The model under review builds one solid part; all positions refer to its coordinate system, in mm. Round coordinates to 2 decimals unless told otherwise and drop trailing zeros. Write each loop counter-clockwise with the first axis right and the second up, starting at its lowest first coordinate (ties: lowest second). Pieces come first, ordered by that corner, then holes. Notation, with made-up numbers: (78, 74.25) - (108, 74.25) arc R21 ccw to (108, 80.25) - close; hole circle Ø11 at (51.5, -11.5). An arc over 180 degrees is marked (long way). Return JSON: item names as keys, results as strings.
Autodesk Inventor part; units mm, degrees
ref_plane "CP_XY" through (0, 0, 0) normal (1, 0, 0) x (0, 0, -1)
ref_plane "CP_YZ" through (0, 0, 0) normal (0, 0, -1) x (0, 1, 0)
ref_plane "CP_ZX" through (0, 0, 0) normal (0, 1, 0) x (1, 0, 0)
sketch "Sketch_1" plane through (0, 0, 0) normal (0, 0, 1) x (1, 0, 0)
  line L0 (0, 0) -> (-4, 0)
  line L1 (-4, 0) -> (-4, 2.0095)
  line L2 (-4, 2.0095) -> (-3.5095, 2.5)
  line L3 (-3.5095, 2.5) -> (-0.75, 2.5)
  line L4 (-0.75, 2.5) -> (0, 1.75)
  line L5 (0, 1.75) -> (0, 0)
  line L6 (0, 0) -> (-4, 0)
revolve "Revolution1" add sketch "Sketch_1" angle 360 about axis through (0, 0, 0) along (1, 0, 0)
thread "Thread1"
sketch "Sketch_2" plane through (-4, 0, 0) normal (-1, 0, 0) x (0, 1, 0)
  line L0 (-1.25, 0.7217) -> (-1.25, -0.7217)
  line L1 (-1.25, -0.7217) -> (0, -1.4434)
  line L2 (0, -1.4434) -> (1.25, -0.7217)
  line L3 (1.25, -0.7217) -> (1.25, 0.7217)
  line L4 (1.25, 0.7217) -> (0, 1.4434)
  line L5 (0, 1.4434) -> (-1.25, 0.7217)
extrude "Extrusion1" cut sketch "Sketch_2" against normal blind 2
sketch "Sketch_3" plane through (0, 0, 0) normal (0, 0, 1) x (1, 0, 0)
  line L0 (-1.2783, 0) -> (-2, 0)
  line L1 (-2, 0) -> (-2, 1.25)
  line L2 (-2, 1.25) -> (-1.2783, 0)
  line L3 (-1.2783, 0) -> (-2, 0)
revolve "Revolution2" cut sketch "Sketch_3" angle 360 about axis through (-1.2783, 0, 0) along (1, 0, 0)
ref_plane "CP_XY" through (0, 0, 0) normal (1, 0, 0) x (0, 0, -1)
ref_plane "CP_YZ" through (0, 0, 0) normal (0, 0, -1) x (0, 1, 0)
ref_plane "CP_ZX" through (0, 0, 0) normal (0, 1, 0) x (1, 0, 0)
properties part number "SET-SCREW5-4"
(1) Mouldability with a two-part tool opening along Y and no side actions: class faces 1 (the cylindrical face through (-2.11, -0.54, -2.44)), 2 (the flat face through (-3.01, 0.63, -1.08)), 3 (the flat face through (0, 0, 0)) as released by +Y, released by -Y, zero draft, split by the parting line, or undercut.
Filled in:
{"face 1": "split by the parting line", "face 2": "undercut", "face 3": "zero draft"}
(2) Add section C-C (x = -1.4). Write out the cut boundary in (y, z), plus the area to 3 significant figures.
Filled in:
{"outline": "circle Ø5 at (0, 0); hole circle Ø0.42 at (0, 0)", "area": "19.5 mm2"}
(3) Add section B-B (x = -0.9). Write out the cut boundary in (y, z).
Filled in:
{"outline": "circle Ø5 at (0, 0)"}
(4) Wall thickness on line 1 (Z direction, x = -3.65, y = 0.6); line 2 (Y direction, x = -3.6, z = 0.8); line 3 (Y direction, x = -2.05, z = 1.35): over which ranges is each line inside the solid? List them lowest first.
Filled in:
{"line 1": "z = -2.28 to -1.1, 1.1 to 2.28", "line 2": "y = -2.27 to -1.11, 1.11 to 2.27", "line 3": "y = -2.1 to -0.16, 0.16 to 2.1"}
(5) Add section A-A (x = -3.15). Write out the cut boundary in (y, z), plus the area to 3 significant figures.
Filled in:
{"outline": "circle Ø5 at (0, 0); hole (-1.25, -0.72) - (0, -1.44) - (1.25, -0.72) - (1.25, 0.72) - (0, 1.44) - (-1.25, 0.72) - close", "area": "14.2 mm2"}
